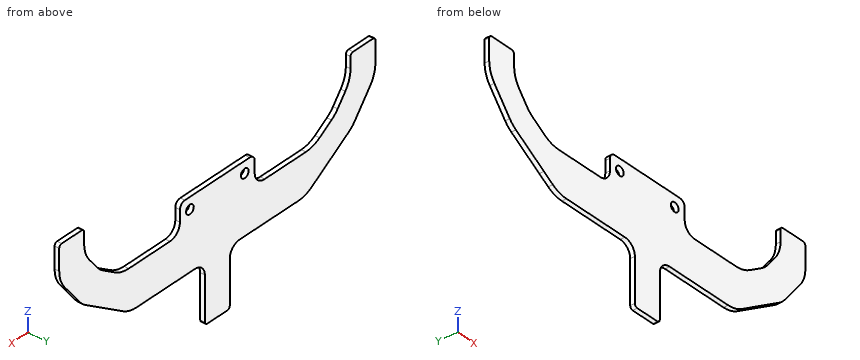
Autodesk Inventor part; units mm, degrees
ref_plane "YZ Plane" through (0, 0, 0) normal (1, 0, 0) x (0, 1, 0)
ref_plane "XZ Plane" through (0, 0, 0) normal (0, 1, 0) x (-1, 0, 0)
ref_plane "XY Plane" through (0, 0, 0) normal (0, 0, 1) x (1, 0, 0)
sketch "Szkic2" plane through (0, 0, 0) normal (0, 1, 0) x (-1, 0, 0)
  line L0 (47.5, 5) -> (-47.5, 5)
  line L1 (-47.5, 5) -> (-47.5, -5)
  line L2 (-47.5, -5) -> (47.5, -5)
  line L3 (47.5, -5) -> (47.5, 5)
  line L4 (47.5, 5) -> (-47.5, -5) construction
  line L5 (-47.5, 5) -> (47.5, -5) construction
  line L6 (0, 24) -> (0, -27)
  point P0 (0, 0)
  dimension "d10" = 10
  dimension "d11" = 95
extrude "Wyciągnięcie proste2" add sketch "Szkic2" along normal blind 1.6
sketch "Szkic3" plane through (0, 1.6, 0) normal (0, 1, 0) x (1, 0, 0)
  line L0 (-47.5, -5) -> (47.5, -5)
  line L1 (47.5, -5) -> (47.5, 5)
  line L2 (47.5, 5) -> (-47.5, 5)
  line L3 (-47.5, 5) -> (-47.5, -5)
  line L4 (52, -8.65) -> (49.4, -5.35) construction
  line L5 (59.75, -18.7) -> (57.1, -15.35) construction
  line L6 (41.3, -1.65) -> (38.65, 1.7) construction
  line L7 (58.425, -17.025) -> (50.7, -7) construction
  line L8 (39.975, 0.025) -> (50.7, -7) construction
  line L9 (58.425, -17.025) -> (58.425, -30) construction
  line L10 (38.5214, -5) -> (47.2545, -10.7203)
  line L11 (47.2545, -10.7203) -> (53.425, -18.728)
  line L12 (53.425, -18.728) -> (53.425, -27.025)
  line L13 (41.5049, 5) -> (54.1455, -3.2797)
  line L14 (54.1455, -3.2797) -> (63.425, -15.322)
  line L15 (63.425, -15.322) -> (63.425, -27.025)
  line L16 (63.425, -27.025) -> (53.425, -27.025)
  line L17 (0, -5) -> (0, 20.232)
  line L18 (-38.5214, -5) -> (-47.2545, -10.7203)
  line L19 (-47.2545, -10.7203) -> (-53.425, -18.728)
  line L20 (-53.425, -18.728) -> (-53.425, -27.025)
  line L21 (-41.5049, 5) -> (-54.1455, -3.2797)
  line L22 (-54.1455, -3.2797) -> (-63.425, -15.322)
  line L23 (-63.425, -15.322) -> (-63.425, -27.025)
  line L24 (-63.425, -27.025) -> (-53.425, -27.025)
  point P0 (0, 0)
  point P1 (-47.5, 1.0732)
  point P2 (47.5, 1.0732)
  dimension "d17" = 5
  dimension "d18" = 5
  dimension "d19" = 10
extrude "Wyciągnięcie proste3" add sketch "Szkic3" against normal up to surface (1.6 mm away) contours L0 L18 L19 L20 L24 L23 L22 L21 L3 | L0 L1 L13 L14 L15 L16 L12 L11 L10
extrude "Wyciągnięcie proste4" cut sketch "Szkic3" against normal through all contours L3 L2 L21 | L2 L1 L13
sketch "Szkic4" plane through (0, 1.6, 0) normal (0, 1, 0) x (1, 0, 0)
  line L0 (-41.5049, 5) -> (-54.1455, -3.2797)
  line L1 (-54.1455, -3.2797) -> (-63.425, -15.322)
  line L2 (-63.425, -15.322) -> (-63.425, -27.025)
  line L3 (-63.425, -27.025) -> (-53.425, -27.025)
  line L4 (-53.425, -27.025) -> (-53.425, -18.728)
  line L5 (-53.425, -18.728) -> (-47.2545, -10.7203)
  line L6 (-47.2545, -10.7203) -> (-38.5214, -5)
  line L7 (-38.5214, -5) -> (38.5214, -5)
  line L8 (38.5214, -5) -> (47.2545, -10.7203)
  line L9 (47.2545, -10.7203) -> (53.425, -18.728)
  line L10 (53.425, -18.728) -> (53.425, -27.025)
  line L11 (53.425, -27.025) -> (63.425, -27.025)
  line L12 (63.425, -27.025) -> (63.425, -15.322)
  line L13 (63.425, -15.322) -> (54.1455, -3.2797)
  line L14 (54.1455, -3.2797) -> (41.5049, 5)
  line L15 (41.5049, 5) -> (-41.5049, 5)
  line L16 (41.5049, 5) -> (35.3982, 9)
  line L17 (35.3982, 9) -> (-35.3982, 9)
  line L18 (-35.3982, 9) -> (-41.5049, 5)
  point P0 (0, 0)
  dimension "d24" = 4
extrude "Wyciągnięcie proste5" add sketch "Szkic4" against normal up to surface (1.6 mm away) contours L18 L17 L16 L15
sketch "Szkic5" plane through (0, 1.6, 0) normal (0, 1, 0) x (1, 0, 0)
  line L0 (-35.3982, 9) -> (-54.1455, -3.2797)
  line L1 (-54.1455, -3.2797) -> (-63.425, -15.322)
  line L2 (-63.425, -15.322) -> (-63.425, -27.025)
  line L3 (-63.425, -27.025) -> (-53.425, -27.025)
  line L4 (-53.425, -27.025) -> (-53.425, -18.728)
  line L5 (-53.425, -18.728) -> (-47.2545, -10.7203)
  line L6 (-47.2545, -10.7203) -> (-38.5214, -5)
  line L7 (-38.5214, -5) -> (38.5214, -5)
  line L8 (38.5214, -5) -> (47.2545, -10.7203)
  line L9 (47.2545, -10.7203) -> (53.425, -18.728)
  line L10 (53.425, -18.728) -> (53.425, -27.025)
  line L11 (53.425, -27.025) -> (63.425, -27.025)
  line L12 (63.425, -27.025) -> (63.425, -15.322)
  line L13 (63.425, -15.322) -> (54.1455, -3.2797)
  line L14 (54.1455, -3.2797) -> (35.3982, 9)
  line L15 (35.3982, 9) -> (-35.3982, 9)
  line L16 (-15, -5) -> (15, -5)
  line L17 (15, -5) -> (15, -15)
  line L18 (15, -15) -> (-15, -15)
  line L19 (-15, -15) -> (-15, -5)
  point P0 (0, 0)
  point P1 (0, -5)
  point P2 (0, 0)
  point P3 (0, -5)
  point P4 (0, -5)
  dimension "d27" = 30
  dimension "d28" = 10
extrude "Wyciągnięcie proste6" add sketch "Szkic5" against normal up to surface (1.6 mm away) contours L7 L17 L18 L19
fillet "Zaokrąglenie1" radius 10 12 edges at (-63.425, 0.8, 15.322) (-54.1455, 0.8, 3.2797) (-35.3982, 0.8, -9) (35.3982, 0.8, -9) (54.1455, 0.8, 3.2797) (63.425, 0.8, 15.322) (-53.425, 0.8, 18.728) (-47.2545, 0.8, 10.7203) (-38.5214, 0.8, 5) (38.5214, 0.8, 5) (47.2545, 0.8, 10.7203) (53.425, 0.8, 18.728)
fillet "Zaokrąglenie2" radius 4 2 edges at (-15, 0.8, 5) (15, 0.8, 5)
fillet "Zaokrąglenie3" radius 2 2 edges at (15, 0.8, 15) (-15, 0.8, 15)
sketch "Szkic6" plane through (0, 1.6, 0) normal (0, 1, 0) x (1, 0, 0)
  line L0 (32.4146, 9) -> (-32.4146, 9)
  line L1 (-5, 9) -> (5, 9)
  line L2 (5, 9) -> (5, 29)
  line L3 (5, 29) -> (-5, 29)
  line L4 (-5, 29) -> (-5, 9)
  point P0 (0, 0)
  point P1 (0, 9)
  point P2 (0, 9)
  dimension "d34" = 10
  dimension "d35" = 20
extrude "Wyciągnięcie proste7" add sketch "Szkic6" against normal up to surface (1.6 mm away)
fillet "Zaokrąglenie4" radius 4 2 edges at (5, 0.8, -9) (-5, 0.8, -9)
fillet "Zaokrąglenie5" radius 1 2 edges at (5, 0.8, -29) (-5, 0.8, -29)
fillet "Zaokrąglenie6" radius 1 4 edges at (-63.425, 0.8, 27.025) (-53.425, 0.8, 27.025) (53.425, 0.8, 27.025) (63.425, 0.8, 27.025)
sketch "Szkic7" plane through (0, 1.6, 0) normal (0, 1, 0) x (1, 0, 0)
  line L0 (-13, -15) -> (13, -15)
  line L1 (15, -13) -> (15, -9)
  line L2 (-15, -9) -> (-15, -13)
  point P0 (0, 0)
  point P1 (-11, -11)
  point P2 (11, -11)
  dimension "d41" = 4
  dimension "d42" = 4
  dimension "d43" = 4
  dimension "d44" = 4
hole "Otwór1" at (-11, 1.6, 11) at (11, 1.6, 11) direction (0, -1, 0) diameter 3.1 depth 15 tip angle 118
properties part number "przód"
Here's how the part is built. I have some questions about the finished solid (model axes, mm). Coordinates: 2 decimals unless noted, no trailing zeros. Order: outer loops, then holes, each group sorted by start corner. A loop starts at its lowest first (then second) coordinate and runs counter-clockwise, first axis right, second up.
Item 1: If we section it at D-D, the plane x = 21.5: List the corners of the cut face in (y, z) for me.
Response values:
outline: (0, -9) - (1.6, -9) - (1.6, 5) - (0, 5) - close
Item 2: If we section it at B-B, the plane z = 20: List the corners of the cut face in (x, y) for me (3 decimals), then the cut area to 3 significant figures.
Response values:
outline: (-63.425, 0) - (-53.195, 0) - (-53.195, 1.6) - (-63.425, 1.6) - close; (53.195, 0) - (63.425, 0) - (63.425, 1.6) - (53.195, 1.6) - close
area: 32.7 mm2
Item 3: I'm going to push flat-ended pins straight in: pin 1 Ø0.5 at (y, z) = (0.5, -20.5) entering from -X; pin 2 Ø4 at (x, z) = (11, 11) entering from +Y; pin 3 Ø0.5 at (y, z) = (1, -24) entering from +X; pin 4 Ø0.5 at (x, y) = (-6, 1) entering from +Z. Where does each tip first touch, or does it pass through?
Response values:
pin 1: stops at x = -5
pin 2: stops at y = 1.6
pin 3: stops at x = 5
pin 4: stops at z = 15
Item 4: I need wall thicknesses on probe 1 along Z at (x, y) = (-11, 0.5); probe 2 along X at (y, z) = (0.5, 11); probe 3 along X at (y, z) = (1, 11.5). Which ranges of each line are inside material? Lowest first, please.
Response values:
probe 1: z = -9 to 9.45, 12.55 to 15
probe 2: x = -60.09 to -47.34, -15 to -12.55, -9.45 to 9.45, 12.55 to 15, 47.34 to 60.09
probe 3: x = -60.48 to -47.82, -15 to -12.47, -9.53 to 9.53, 12.47 to 15, 47.82 to 60.48
Item 5: If we section it at C-C, the plane y = 0.8: Give the number of separate pieces and of enclosed holes in the cut face, then the cut area to 3 significant figures.
Response values:
separate pieces: 1
enclosed holes: 2
area: 2,310 mm2
Item 6: If we section it at A-A, the plane x = -11: List the corners of the cut face in (y, z) for me.
Response values:
outline: (0, -9) - (1.6, -9) - (1.6, 9.45) - (0, 9.45) - close; (0, 12.55) - (1.6, 12.55) - (1.6, 15) - (0, 15) - close
